Answer from the drawing. Dimensions are ordinates in mm from the lowest x, y and z of the part. A direction names the side the tool comes from. Coordinates: 2 decimals unless noted, no trailing zeros. Order: outer loops, then holes, each group sorted by start corner. A loop starts at its lowest first (then second) coordinate and runs counter-clockwise, first axis right, second up.
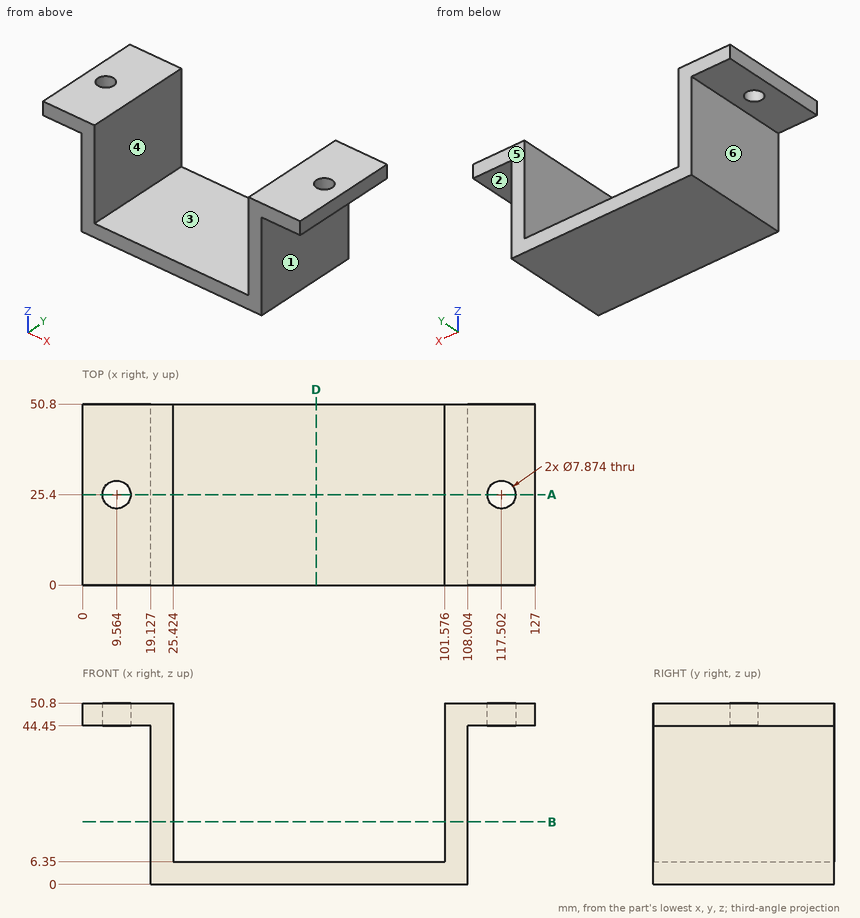
1) Section B-B (z = 17.5) is taken. Give the vertices of the cut face in (x, y) (1 decimal).
2) Section A-A (y = 25.4) is taken. Give the number of separate pieces and of enclosed holes in the cut face, then the cut area to 3 significant figures.
3) Determine the mould class of the marked faces 1, 2 and 3 for opening direction X: released by +X, released by -X, zero draft, split by the parting line, or undercut.
4) Consider L1, parallel to X at y = 25, z = 46 (1 decimal); L2, parallel to X at y = 29.5, z = 48.5 (1 decimal); L3, parallel to X at y = 14, z = 12 (1 decimal). Determine where each line is inside the solid, lowest interval first.
5) Section D-D (x = 65.5) is taken. Give the vertices of the cut face in (y, z).
6) A tool of negligible diameter and unlimited length cuts with its end or side. For the marked faces 4, 5 and 6, from which of +Z, -Z, +X, -X, +Y, -Y can it reach the whole face along a straight path? Write none if from no direction.
7) Each of these flat-tipped pins is pushed along its axis until it touches: P1, Ø22, axis at y = 34.5, z = 14.5, coming from the -X side; P2, Ø1.5, axis at y = 16.5, z = 34.5, coming from the +X side; P3, Ø10, axis at x = 114, y = 34.5, coming from the -Z side; P4, Ø6.5, axis at x = 9.56, y = 25.4, coming from the +Z side. Where does it stop, or does it pass through?
Filled sheet:
1. outline: (19.1, 0) - (25.4, 0) - (25.4, 50.8) - (19.1, 50.8) - close; (101.6, 0) - (108, 0) - (108, 50.8) - (101.6, 50.8) - close
2. separate pieces: 3
2. enclosed holes: 0
2. area: 1,270 mm2
3. face 1: released by +X
3. face 2: zero draft
3. face 3: undercut
4. L1: x = 0 to 5.6, 13.5 to 25.4, 101.6 to 113.6, 121.4 to 127
4. L2: x = 0 to 25.4, 101.6 to 127
4. L3: x = 19.1 to 25.4, 101.6 to 108
5. outline: (0, 0) - (50.8, 0) - (50.8, 6.35) - (0, 6.35) - close
6. face 4: +Z, +Y, -Y
6. face 5: +Z, -Z, +X, -X, +Y
6. face 6: -Z, -X, +Y, -Y
7. P1: stops at x = 19.13
7. P2: stops at x = 108
7. P3: stops at z = 44.45
7. P4: passes through
